```python
from build123d import *

# Parameters (mm, degrees)
CYLINDER023_R            = 1.75
CYLINDER023_DEPTH        = 80
CYLINDER023_PITCH_ANGLE  = 90
CYLINDER022_R            = 1.75
CYLINDER022_DEPTH        = 80
CYLINDER022_PITCH_ANGLE  = 90
BOX017_W                 = 134
BOX017_H                 = 14
BOX017_DEPTH             = 4
BOX017_PLACEMENT_ANGLE   = 90
PAD026_DEPTH             = 20
CLONE137_PLACEMENT_ANGLE = 180
BOX015_W                 = 400
BOX015_H                 = 400
BOX015_DEPTH             = 185
BOX016_W                 = 134
BOX016_H                 = 14
BOX016_DEPTH             = 4


with BuildPart() as cilindro019:
    # Cylinder023 → Cylinder023 (new body)
    with BuildSketch(Plane.XY):
        Circle(CYLINDER023_R)
    extrude(amount=CYLINDER023_DEPTH)


with BuildPart() as cilindro019_1:
    # Cylinder023 pitch: moved
    add(cilindro019.part.rotate(Axis((0, 0, 0), (0, 1, 0)), CYLINDER023_PITCH_ANGLE))


with BuildPart() as cilindro019_2:
    # Cylinder023 placement: moved
    add(cilindro019_1.part.moved(Location((-40, -5.5, 37.5))))


with BuildPart() as fusion024:
    # Cylinder022 → Cylinder022 (new body)
    with BuildSketch(Plane.XY):
        Circle(CYLINDER022_R)
    extrude(amount=CYLINDER022_DEPTH)


with BuildPart() as fusion024_1:
    # Cylinder022 pitch: moved
    add(fusion024.part.rotate(Axis((0, 0, 0), (0, 1, 0)), CYLINDER022_PITCH_ANGLE))


with BuildPart() as fusion024_2:
    # Cylinder022 placement: moved
    add(fusion024_1.part.moved(Location((-40, 5.5, 37.5))))

    # Fusion024: union Cilindro019
    add(cilindro019_2.part)


with BuildPart() as cubo017:
    # Box017 → Box017 (new body)
    with BuildSketch(Plane.XY):
        with Locations((67, 7)):
            Rectangle(BOX017_W, BOX017_H)
    extrude(amount=BOX017_DEPTH)


with BuildPart() as cubo017_1:
    # Box017 placement: moved
    add(cubo017.part.moved(Location((7, -67, 47))).rotate(Axis((7, -67, 47), (0, 0, 1)), BOX017_PLACEMENT_ANGLE))


with BuildPart() as pad026:
    # Sketch024 → Pad026 (new body)
    with BuildSketch(Plane.XZ.offset(10)):
        Polygon((-25.98196, 33.981216), (-30.98196, 33.981216), (-30.98196, 75.756836), (-25.98196, 77.981216), align=None)
    extrude(amount=-PAD026_DEPTH)


with BuildPart() as clone_of_pad026:
    # Clone137 base: copy of Pad026
    add(pad026.part)


with BuildPart() as clone_of_pad026_1:
    # Clone137 placement: moved
    add(clone_of_pad026.part.moved(Location((0, 0, 0))).rotate(Axis((0, 0, 0), (0, 0, 1)), CLONE137_PLACEMENT_ANGLE))


with BuildPart() as esfera001:
    # Sphere001 → Sphere001 (revolve)
    with BuildSketch(Plane.XZ):
        with BuildLine():
            ThreePointArc((0, -82), (82, 0), (0, 82))
            Line((0, 82), (0, -82))
        make_face()
    revolve(axis=Axis((0, 0, 0), (0, 0, 1)))


with BuildPart() as cubo015:
    # Box015 → Box015 (new body)
    with BuildSketch(Plane(origin=(-200, -200, -150), x_dir=(1, 0, 0), z_dir=(0, 0, 1))):
        with Locations((200, 200)):
            Rectangle(BOX015_W, BOX015_H)
    extrude(amount=BOX015_DEPTH)


with BuildPart() as cut034:
    # Sphere → Sphere (revolve)
    with BuildSketch(Plane.XZ):
        with BuildLine():
            ThreePointArc((0, -85), (85, 0), (0, 85))
            Line((0, 85), (0, -85))
        make_face()
    revolve(axis=Axis((0, 0, 0), (0, 0, 1)))

    # Cut033: cut Cubo015
    add(cubo015.part, mode=Mode.SUBTRACT)

    # Cut034: cut Esfera001
    add(esfera001.part, mode=Mode.SUBTRACT)


with BuildPart() as cut035:
    # Box016 → Box016 (new body)
    with BuildSketch(Plane(origin=(-67, -7, 47), x_dir=(1, 0, 0), z_dir=(0, 0, 1))):
        with Locations((67, 7)):
            Rectangle(BOX016_W, BOX016_H)
    extrude(amount=BOX016_DEPTH)

    # Fusion023: union Cubo017, Pad026, Clone of Pad026, Cut034
    add(cubo017_1.part)
    add(pad026.part)
    add(clone_of_pad026_1.part)
    add(cut034.part)

    # Cut035: cut Fusion024
    add(fusion024_2.part, mode=Mode.SUBTRACT)


solid = cut035.part
```
Part model, mm, in its own coordinate system. A direction names the side the tool comes from. Coordinates: 2 decimals unless noted, no trailing zeros. Order: outer loops, then holes, each group sorted by start corner. A loop starts at its lowest first (then second) coordinate and runs counter-clockwise, first axis right, second up. Notation, with made-up numbers: (55, 25) - (114, 25) arc R4 cw to (114, 32) - close; hole circle Ø8 at (-16.75, -2.5). An arc over 180 degrees is marked (long way). Return JSON: item names as keys, results as strings. Group by question number.
Item 1: Which spindle directions (+Z, -Z, +X, -X, +Y, -Y) get a long thin tool onto all of the face, cutting with end or side? Do faces 4 (the face through (28.447, -6.17, 35.883)), 5 (the face through (-17, -7, 49)). Say none if no direction does.
Item 2: Drill centre lines: probe 1 along X at (y, z) = (4, 46.5); probe 2 along Y at (x, z) = (28.65, 37.5); probe 3 along Y at (x, z) = (27, 37). Where is each one in solid material? Low to high. Write a range as from..to.
Item 3: Cut at A-A (z = 60). List the corners of the cut face in (x, y), plus the area to 3 significant figures.
Item 4: Cut at B-B (y = -42.5). List the corners of the cut face in (x, z), plus the area to 3 significant figures.
Item 5: Pull direction Y, two halves, no side cores. Call faces 1 (the face through (49, -7, 49)), 2 (the face through (-25.982, 0, 56)), 3 (the face through (63, -40, 35)): pulls with the +Y half, pulls with the -Y half, needs draft (parallel to the pull), parting line crosses it, or undercut.
Item 6: Cut at C-C (x = 47). List the corners of the cut face in (y, z).
Item 7: Pin check, flat tips, straight feed: pin 1 (6 mm diameter, centred on x = 43, z = 46, fed in from -Y); pin 2 (15.5 mm diameter, centred on x = 42, y = 1.5, fed in from -Z); pin 3 (12 mm diameter, centred on x = 60, y = -45.5, fed in from -Z); pin 4 (2 mm diameter, centred on y = 36, z = 78.5, fed in from +X). Stop position of each tip, or through.
Check values:
{
 "1": {"face 4": "none", "face 5": "-Z"},
 "2": {"probe 1": "x = -71.04..-67.42, -30.98..-25.98, 25.98..30.98, 67.42..71.04", "probe 2": "y = -70.7..-67.06, -10..-7.25, -3.75..3.75, 7.25..10, 67.06..70.7", "probe 3": "y = -71.6..-68.01, -10..-7.18, -3.82..3.82, 7.18..10, 68.01..71.6"},
 "3": {"outline": "circle Ø120.42 at (0, 0); (-30.98, -10) - (-25.98, -10) - (-25.98, 10) - (-30.98, 10) - close; (25.98, -10) - (30.98, -10) - (30.98, 10) - (25.98, 10) - close; hole circle Ø111.79 at (0, 0)", "area": "1,770 mm2"},
 "4": {"outline": "(-64.76, 35) - (-60.77, 35) arc R70.13 cw to (60.77, 35) - (64.76, 35) arc R73.61 ccw to start; (-7, 47) - (7, 47) - (7, 51) - (-7, 51) - close", "area": "588 mm2"},
 "5": {"face 1": "undercut", "face 2": "undercut", "face 3": "needs draft"},
 "6": {"outline": "(-61.57, 35) - (-57.36, 35) arc R67.19 cw to (57.36, 35) - (61.57, 35) arc R70.82 ccw to start; (-7, 47) - (7, 47) - (7, 51) - (-7, 51) - close"},
 "7": {"pin 1": "stops at y = -60.24", "pin 2": "stops at z = 47", "pin 3": "stops at z = 35", "pin 4": "passes through"}
}
